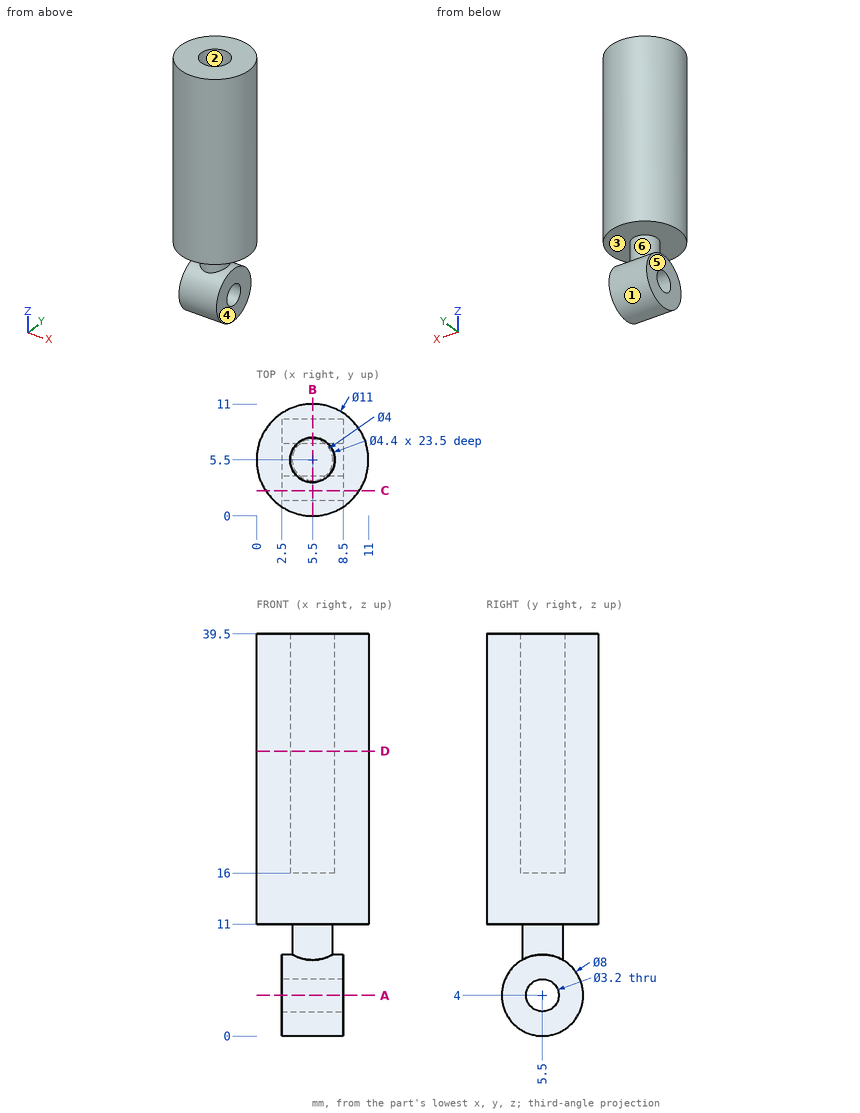
Print and shaded views of the part. All mm, measured from the part's lowest x, y and z. A direction names the side the tool comes from. Coordinates: 2 decimals unless noted, no trailing zeros. Write each loop counter-clockwise with the first axis right and the second up, starting at its lowest first coordinate (ties: lowest second). Pieces come first, ordered by that corner, then holes.
(1) Two-plate mould, pull along Y, no slides. Class the marked faces 1, 2 and 3: +Y half, -Y half, draft (parallel to the pull), parting line (faces both ways), or undercut.
(2) Drill centre lines: probe 1 along Z at (x, y) = (4.55, 5.5); probe 2 along Y at (x, z) = (5.5, 32.25); probe 3 along Z at (x, y) = (2.75, 6). Where is each one in solid material? Low to high.
(3) 3-axis set-ups, long thin cutter, end or side, ignore diameter. For the marked faces 4, 5 and 6: which of +Z, -Z, +X, -X, +Y, -Y reach the whole face in a straight line?
(4) Cut at B-B, the plane x = 5.5. List the corners of the cut face in (y, z).
(5) Flat gauge pins, fed straight in: pin 1 (6 mm diameter, centred on y = 2, z = 33.5, fed in from +X); pin 2 (5 mm diameter, centred on y = 5.5, z = 4, fed in from -X); pin 3 (5 mm diameter, centred on x = 2.5, y = 9.5, fed in from -Z). Where does each tip first touch, or does it go through?
(6) Cut at C-C, the plane y = 2.5. List the corners of the cut face in (x, z), and give its area (3 significant figures).
(7) Cut at A-A, the plane z = 4. List the corners of the cut face in (x, y), and give its area (3 significant figures).
(8) Cut at D-D, the plane z = 28. List the corners of the cut face in (x, y), and give its area (3 significant figures).
Geometry says:
1. face 1: parting line
1. face 2: undercut
1. face 3: draft
2. probe 1: z = 0 to 2.4, 5.6 to 16
2. probe 2: y = 0 to 3.3, 7.7 to 11
2. probe 3: z = 0.03 to 2.48, 5.52 to 7.97, 11 to 39.5
3. face 4: -Z, +X, +Y, -Y
3. face 5: -Z, -X, +Y, -Y
3. face 6: none
4. outline: (0, 11) - (3.5, 11) - (3.5, 7.46) arc R4 ccw (long way) to (7.5, 7.46) - (7.5, 11) - (11, 11) - (11, 39.5) - (7.7, 39.5) - (7.7, 16) - (3.3, 16) - (3.3, 39.5) - (0, 39.5) - close; hole circle Ø3.2 at (5.5, 4)
5. pin 1: stops at x = 10.98
5. pin 2: stops at x = 2.5
5. pin 3: stops at z = 0.29
6. outline: (0.89, 11) - (10.11, 11) - (10.11, 39.5) - (0.89, 39.5) - close; (2.5, 1.35) - (8.5, 1.35) - (8.5, 6.65) - (2.5, 6.65) - close
6. area: 295 mm2
7. outline: (2.5, 1.5) - (8.5, 1.5) - (8.5, 3.9) - (2.5, 3.9) - close; (2.5, 7.1) - (8.5, 7.1) - (8.5, 9.5) - (2.5, 9.5) - close
7. area: 28.8 mm2
8. outline: circle Ø11 at (5.5, 5.5); hole circle Ø4.4 at (5.5, 5.5)
8. area: 79.8 mm2
